Check sheet for the modelled part. Datum: model origin and axes. Units: mm. Face numbers are marked on the shaded views. A direction names the side the tool comes from. Give positions to 0.01 mm unless a question says otherwise; leave off trailing zeros. Loops run counter-clockwise (first coordinate to the right, second up) from the corner with the lowest first, then second, coordinate; pieces in that order, holes last. Notation, with made-up numbers: M -21,75 L 13,75 A27 ccw 13,114 Z; hole C -16,-11 d10. An arc over 180 degrees is marked long. Put each result on its own line as item: value. Start each with the question number.
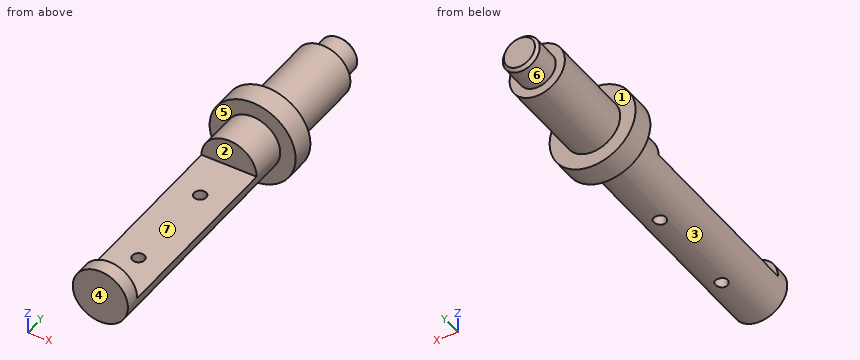
```python
from build123d import *

# Parameters (mm, degrees)
SKETCH1_R           = 28
BOSS_EXTRUDE1_DEPTH = 118.7
SKETCH3_R           = 43.6
BOSS_EXTRUDE2_DEPTH = 24
SKETCH4_R           = 28
SKETCH4_R_2         = 18.75
CUT_EXTRUDE1_DEPTH  = 28.9
CHAMFER1_SIZE       = 3
SKETCH6_R           = 28
BOSS_EXTRUDE3_DEPTH = 38.2
BOSS_EXTRUDE4_DEPTH = 193.8
SKETCH9_R           = 28
BOSS_EXTRUDE5_DEPTH = 15.1
SKETCH10_R          = 6.25
CUT_EXTRUDE2_DEPTH  = 28.1


with BuildPart() as part:
    # Sketch1 → Boss-Extrude1 (new body)
    with BuildSketch(Plane(origin=(0, 0, 0), x_dir=(1, 0, 0), z_dir=(0, 1, 0))):
        Circle(SKETCH1_R)
    extrude(amount=-BOSS_EXTRUDE1_DEPTH)

    # Sketch3 → Boss-Extrude2 (add)
    with BuildSketch(Plane.XZ.offset(118.7)):
        Circle(SKETCH3_R)
    extrude(amount=BOSS_EXTRUDE2_DEPTH)

    # Sketch4 → Cut-Extrude1 (cut)
    with BuildSketch(Plane(origin=(0, 0, 0), x_dir=(1, 0, 0), z_dir=(0, 1, 0))):
        Circle(SKETCH4_R)
        Circle(SKETCH4_R_2, mode=Mode.SUBTRACT)
    extrude(amount=-CUT_EXTRUDE1_DEPTH, mode=Mode.SUBTRACT)

    # Chamfer1
    chamfer1_edges = [part.edges().sort_by_distance(p)[0] for p in [
        (-18.75, 0, 0),
    ]]
    chamfer(chamfer1_edges, length=CHAMFER1_SIZE)

    # Sketch6 → Boss-Extrude3 (add)
    with BuildSketch(Plane.XZ.offset(142.7)):
        Circle(SKETCH6_R)
    extrude(amount=BOSS_EXTRUDE3_DEPTH)

    # Sketch8 → Boss-Extrude4 (add)
    with BuildSketch(Plane.XZ.offset(180.9)):
        with BuildLine():
            Line((-28, 0), (28, 0))
            ThreePointArc((28, 0), (0, -28), (-28, 0))
        make_face()
    extrude(amount=BOSS_EXTRUDE4_DEPTH)

    # Sketch9 → Boss-Extrude5 (add)
    with BuildSketch(Plane.XZ.offset(374.7)):
        Circle(SKETCH9_R)
    extrude(amount=BOSS_EXTRUDE5_DEPTH)

    # Sketch10 → Cut-Extrude2 (cut)
    with BuildSketch(Plane.XY):
        with Locations((0, -227.8)):
            Circle(SKETCH10_R)
        with Locations((0, -327.8)):
            Circle(SKETCH10_R)
    extrude(amount=-CUT_EXTRUDE2_DEPTH, mode=Mode.SUBTRACT)


solid = part.part
```
Q1. Access from +Z, -Z, +X, -X, +Y, -Y to the whole of each face (thin tool, end or side, straight path). Record for the marked faces 4, 5, 6 and 7.
Q2. Depth check by flat-ended pin: P1, Ø6, axis at y = -157, z = -18.5, coming from the -X side; P2, Ø1, axis at y = -119.5, z = 2, coming from the -X side; P3, Ø14.5, axis at x = 0, y = -227.8, coming from the -Z side; P4, Ø8.5, axis at x = 3.5, z = 18.5, coming from the +Y side. Enter the tip coordinate at first touch or a pass-through.
Q3. Section check D-D, the plane z = -37.5. Record the cut outline in (x, y).
Q4. Thickness scan on line 1 along Y through (x, z) = (0, -12); line 2 along Y through (x, z) = (0, -21); line 3 along Y through (x, z) = (-4.5, 15). Record the ranges inside material, lowest first. Write a range as [from, to].
Q5. Section check A-A, the plane x = 0. Give the number of separate pieces and of enclosed holes in the cut face, then the cut area to 3 significant figures.
Q6. Mould release check, pull along Y, two halves, no side actions. Record for the marked faces 1, 2 and 3: pulls with the +Y half, pulls with the -Y half, needs draft (parallel to the pull), parting line crosses it, or undercut.
Q7. Section check B-B, the plane y = -227.8. Record the cut outline in (x, z), then the cut area to 3 significant figures.
Q8. Section check C-C, the plane y = -101.5. Record the cut outline in (x, z), then the cut area to 3 significant figures.
Found:
1. face 4: +Z, -Z, +X, -X, -Y
1. face 5: -Y
1. face 6: +Y
1. face 7: +Z, +X, -X
2. P1: stops at x = -23.32
2. P2: stops at x = -43.57
2. P3: stops at z = -28
2. P4: stops at y = 0
3. outline: M -22.24,-142.7 L 22.24,-142.7 L 22.24,-118.7 L -22.24,-118.7 Z
4. line 1: y = [-389.8, -334.05], [-321.55, -234.05], [-221.55, 0]
4. line 2: y = [-389.8, -334.05], [-321.55, -234.05], [-221.55, -28.9]
4. line 3: y = [-389.8, -374.7], [-180.9, 0]
5. separate pieces: 3
5. enclosed holes: 0
5. area: 15,900 mm^2
6. face 1: pulls with the +Y half
6. face 2: undercut
6. face 3: needs draft
7. outline: M -28,0 A28 ccw -6.25,-27.29 L -6.25,0 Z; M 6.25,-27.29 A28 ccw 28,0 L 6.25,0 Z
7. area: 884 mm^2
8. outline: C 0,0 d56
8. area: 2,460 mm^2
